from build123d import *

# Parameters (mm, degrees)
SKETCH1_W           = 60
SKETCH1_H           = 60
SKETCH1_R           = 10
BOSS_EXTRUDE1_DEPTH = 60
SKETCH2_W           = 10
SKETCH2_H           = 60
BOSS_EXTRUDE2_DEPTH = 60
FILLET1_R           = 2


with BuildPart() as part:
    # Sketch1 → Boss-Extrude1 (new body)
    with BuildSketch(Plane.XY):
        with Locations((30, 30)):
            Rectangle(SKETCH1_W, SKETCH1_H)
        with Locations((30, 30)):
            Circle(SKETCH1_R, mode=Mode.SUBTRACT)
    extrude(amount=BOSS_EXTRUDE1_DEPTH)

    # Sketch2 → Boss-Extrude2 (add)
    with BuildSketch(Plane(origin=(60, 0, 0), x_dir=(0, 0, -1), z_dir=(1, 0, 0))):
        with Locations((-5, 30)):
            Rectangle(SKETCH2_W, SKETCH2_H)
    extrude(amount=BOSS_EXTRUDE2_DEPTH)

    # Fillet1
    fillet1_edges = [part.edges().sort_by_distance(p)[0] for p in [
        (20, 30, 0),
        (20, 30, 60),
        (60, 30, 60),
        (30, 60, 60),
        (60, 30, 10),
        (90, 60, 10),
        (90, 0, 10),
        (120, 30, 0),
        (120, 60, 5),
        (120, 30, 10),
        (120, 0, 5),
        (0, 30, 60),
        (60, 60, 0),
        (60, 0, 0),
        (0, 30, 0),
        (0, 60, 30),
        (60, 60, 35),
        (60, 0, 35),
        (0, 0, 30),
        (30, 0, 60),
    ]]
    fillet(fillet1_edges, radius=FILLET1_R)


solid = part.part
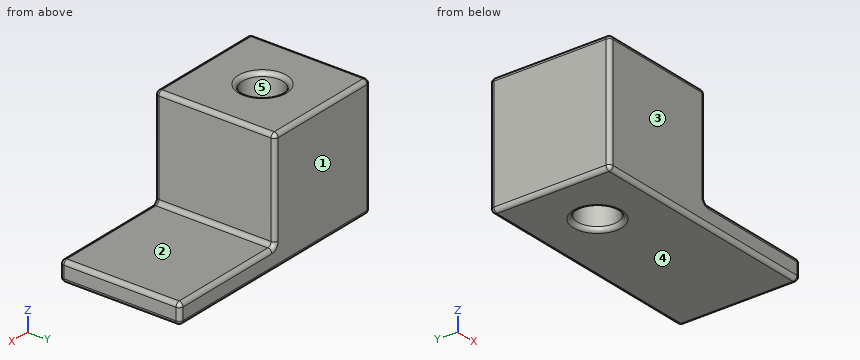
Input: part model. Units: mm. Frame: model coordinates. Face numbers are marked on the shaded views. A direction names the side the tool comes from. Give positions to 0.01 mm unless a question says otherwise; leave off trailing zeros. Loops run counter-clockwise (first coordinate to the right, second up) from the corner with the lowest first, then second, coordinate; pieces in that order, holes last. Notation, with made-up numbers: M -23.75,45.5 L 26.25,45.5 A20 cw 26.25,52.5 Z; hole C -3,-34.75 d8. An arc over 180 degrees is marked long. Use CSV: the item, a comma, the result in double quotes.
(1) Section C-C, the plane z = 5. Return loops of the section in (x, y), plus the area to 3 significant figures.
Outcome:
outline,"M 0,2 A2 ccw 2,0 L 118,0 A2 ccw 120,2 L 120,58 A2 ccw 118,60 L 2,60 A2 ccw 0,58 Z; hole C 30,30 d20"
area,"6,880 mm²"
(2) Pull-direction query (Y, two-part tool) for the marked faces 3, 4 and 5; classes: pulls with the +Y half, pulls with the -Y half, needs draft (parallel to the pull), parting line crosses it, or undercut.
Outcome:
face 3,"pulls with the -Y half"
face 4,"needs draft"
face 5,"undercut"
(3) Material intervals for L1, parallel to X at y = 49.5, z = 43; L2, parallel to Z at x = 94.5, y = 51; L3, parallel to Y at x = 30, z = 25, sorted ascending. Write a range as [from, to].
Outcome:
L1,"x = [0, 60]"
L2,"z = [0, 10]"
L3,"y = [0, 20], [40, 60]"
(4) Pin query (flat end, axial travel): P1, Ø23, axis at y = 42.5, z = 33.5, coming from the +X side. Return the tip coordinate at first contact, or that it passes through.
Outcome:
P1,"stops at x = 60"
(5) Set-up query: the marked faces 1 and 2. Return all of +Z, -Z, +X, -X, +Y, -Y with unobstructed straight access to the full face (end or side cutting, diameter ignored); none if empty.
Outcome:
face 1,"+Z, -Z, +X, -X, +Y"
face 2,"+Z, +X, +Y, -Y"
(6) Section A-A, the plane y = 30. Return loops of the section in (x, z).
Outcome:
outline,"M 0,2 A2 ccw 2,0 L 18,0 A2 ccw 20,2 L 20,58 A2 ccw 18,60 L 2,60 A2 ccw 0,58 Z; M 40,2 A2 ccw 42,0 L 118,0 A2 ccw 120,2 L 120,8 A2 ccw 118,10 L 62,10 A2 cw 60,12 L 60,58 A2 ccw 58,60 L 42,60 A2 ccw 40,58 Z"
(7) Section D-D, the plane x = 95. Return loops of the section in (y, z), plus the area to 3 significant figures.
Outcome:
outline,"M 0,2 A2 ccw 2,0 L 58,0 A2 ccw 60,2 L 60,8 A2 ccw 58,10 L 2,10 A2 ccw 0,8 Z"
area,"597 mm²"
(8) Section B-B, the plane x = 30. Return loops of the section in (y, z), plus the area to 3 significant figures.
Outcome:
outline,"M 0,2 A2 ccw 2,0 L 18,0 A2 ccw 20,2 L 20,58 A2 ccw 18,60 L 2,60 A2 ccw 0,58 Z; M 40,2 A2 ccw 42,0 L 58,0 A2 ccw 60,2 L 60,58 A2 ccw 58,60 L 42,60 A2 ccw 40,58 Z"
area,"2,390 mm²"
